Build history of the part. All positions in model axes, mm. A direction names the side the tool comes from. Give positions to 0.01 mm unless a question says otherwise; leave off trailing zeros. One line per question, with ' | ' between items. Start each with the question number.
(1) Drill centre lines: L1, parallel to Z at x = 156, y = 66; L2, parallel to Y at x = 9.5, z = 3.5; L3, parallel to X at y = 36, z = 3.75. Where is each one in solid material? Low to high. Write a range as from..to.
(2) 3-axis set-ups, long thin cutter, end or side, ignore diameter. For faces 4 (the face through (5.427, 67.216, 5.115)), 5 (the face through (154.573, 64.784, 5.115)), 6 (the face through (79, 0, 4)): which of +Z, -Z, +X, -X, +Y, -Y reach the whole face in a straight line?
(3) Flat gauge pins, fed straight in: pin 1 Ø2.5 at (y, z) = (6, 4) entering from -X; pin 2 Ø2 at (y, z) = (36, 4) entering from +X; pin 3 Ø3 at (y, z) = (36, 4) entering from +X. Where does each tip first touch, or does it go through?
(4) Mould opens along Z. For faces 1 (the face through (12, 6, 4)), 2 (the face through (160, 35, 2)), 3 (the face through (79, 37, 0)) say: pulls with the +Z half, pulls with the -Z half, needs draft (parallel to the pull), parting line crosses it, or undercut.
```python
from build123d import *

# Parameters (mm, degrees)
BOX_W          = 160
BOX_H          = 72
BOX_DEPTH      = 8
SKETCH_R       = 1.65
HOLE_DEPTH     = 11.00858
HOLE_TIPS_R    = 1.65
SKETCH001_R    = 1.65
HOLE001_DEPTH  = 11.00858
HOLE001_TIPS_R = 1.65


with BuildPart() as part:
    # Box → Box (new body)
    with BuildSketch(Plane.XY):
        with Locations((80, 36)):
            Rectangle(BOX_W, BOX_H)
    extrude(amount=BOX_DEPTH)

    # Sketch (on Face1 of BaseFeature) → Hole (cut)
    with BuildSketch(Plane(origin=(0, 0, 0), x_dir=(0, -1, 0), z_dir=(-1, 0, 0))):
        with Locations((-66, 4)):
            Circle(SKETCH_R)
        with Locations((-36, 4)):
            Circle(SKETCH_R)
        with Locations((-6, 4)):
            Circle(SKETCH_R)
    extrude(amount=-HOLE_DEPTH, mode=Mode.SUBTRACT)

    # Hole tips → Hole tip 1 section 0
    with BuildSketch(Plane(origin=(11.00858, 0, 0), x_dir=(0, -1, 0), z_dir=(-1, 0, 0)), mode=Mode.PRIVATE) as hole_tip_1_s0:
        with Locations((-66, 4)):
            Circle(HOLE_TIPS_R)
    loft([hole_tip_1_s0.sketch, Vertex(12, 66, 4)], mode=Mode.SUBTRACT)

    # Hole tips → Hole tip 2 section 0
    with BuildSketch(Plane(origin=(11.00858, 0, 0), x_dir=(0, -1, 0), z_dir=(-1, 0, 0)), mode=Mode.PRIVATE) as hole_tip_2_s0:
        with Locations((-36, 4)):
            Circle(HOLE_TIPS_R)
    loft([hole_tip_2_s0.sketch, Vertex(12, 36, 4)], mode=Mode.SUBTRACT)

    # Hole tips → Hole tip 3 section 0
    with BuildSketch(Plane(origin=(11.00858, 0, 0), x_dir=(0, -1, 0), z_dir=(-1, 0, 0)), mode=Mode.PRIVATE) as hole_tip_3_s0:
        with Locations((-6, 4)):
            Circle(HOLE_TIPS_R)
    loft([hole_tip_3_s0.sketch, Vertex(12, 6, 4)], mode=Mode.SUBTRACT)

    # Sketch001 (on Face9 of Hole) → Hole001 (cut)
    with BuildSketch(Plane.YZ.offset(160)):
        with Locations((6, 4)):
            Circle(SKETCH001_R)
        with Locations((36, 4)):
            Circle(SKETCH001_R)
        with Locations((66, 4)):
            Circle(SKETCH001_R)
    extrude(amount=-HOLE001_DEPTH, mode=Mode.SUBTRACT)

    # Hole001 tips → Hole001 tip 1 section 0
    with BuildSketch(Plane.YZ.offset(148.99142), mode=Mode.PRIVATE) as hole001_tip_1_s0:
        with Locations((6, 4)):
            Circle(HOLE001_TIPS_R)
    loft([hole001_tip_1_s0.sketch, Vertex(148, 6, 4)], mode=Mode.SUBTRACT)

    # Hole001 tips → Hole001 tip 2 section 0
    with BuildSketch(Plane.YZ.offset(148.99142), mode=Mode.PRIVATE) as hole001_tip_2_s0:
        with Locations((36, 4)):
            Circle(HOLE001_TIPS_R)
    loft([hole001_tip_2_s0.sketch, Vertex(148, 36, 4)], mode=Mode.SUBTRACT)

    # Hole001 tips → Hole001 tip 3 section 0
    with BuildSketch(Plane.YZ.offset(148.99142), mode=Mode.PRIVATE) as hole001_tip_3_s0:
        with Locations((66, 4)):
            Circle(HOLE001_TIPS_R)
    loft([hole001_tip_3_s0.sketch, Vertex(148, 66, 4)], mode=Mode.SUBTRACT)


solid = part.part
```
Final values:
1) L1: 0..2.35, 5.65..8 | L2: 0..4.43, 7.57..34.43, 37.57..64.43, 67.57..72 | L3: 11.85..148.15
2) face 4: -X | face 5: +X | face 6: +Z, -Z, +X, -X, -Y
3) pin 1: x = 11.25 | pin 2: x = 148.6 | pin 3: x = 148.9
4) face 1: undercut | face 2: needs draft | face 3: pulls with the -Z half
